```python
from build123d import *

# Parameters (mm, degrees)
SKETCH1_R               = 9
SKETCH1_W               = 9.9
SKETCH1_H               = 9.9
BOSS_EXTRUDE1_DEPTH     = 10
SKETCH2_R               = 17.5
BOSS_EXTRUDE2_DEPTH     = 6.5
CUT_EXTRUDE1_REACH      = 28.693
SKETCH3_R               = 1.25
CUT_EXTRUDE2_DEPTH      = 30.744747435
CUT_EXTRUDE2_DEPTH_BACK = 30.744747435
SKETCH4_R               = 1.5
CUT_EXTRUDE3_DEPTH      = 10
CUT_EXTRUDE3_DEPTH_BACK = 10
SKETCH6_W               = 9.9
SKETCH6_H               = 9.9
SKETCH8_W               = 5.75
SKETCH8_H               = 2.75
CUT_EXTRUDE4_DEPTH      = 5
CUT_EXTRUDE5_DEPTH      = 2.75
CIRPATTERN1_START       = 11.875
CIRPATTERN1_OUTLINE_R   = 1.25
CIRPATTERN1_DEPTH       = 2.75


# Read off the part's stored shape, not the designer's step: CirPattern1
with BuildPart() as part:
    # Sketch1 → Boss-Extrude1 (new body)
    with BuildSketch(Plane(origin=(0, 0, 0), x_dir=(1, 0, 0), z_dir=(0, 1, 0))):
        with Locations(Location((0, 0, 0), (0, 0, 270))):
            Circle(SKETCH1_R)
        Rectangle(SKETCH1_W, SKETCH1_H, mode=Mode.SUBTRACT)
    extrude(amount=BOSS_EXTRUDE1_DEPTH)

    # Sketch2 → Boss-Extrude2 (add)
    with BuildSketch(Plane(origin=(0, 10, 0), x_dir=(1, 0, 0), z_dir=(0, 1, 0))):
        with Locations(Location((0, 0, 0), (0, 0, 90))):
            Circle(SKETCH2_R)
    extrude(amount=BOSS_EXTRUDE2_DEPTH)

    # Sketch3 → Cut-Extrude1 (cut, up to next)
    with BuildSketch(Plane.XZ.offset(-10), mode=Mode.PRIVATE) as cut_extrude1_sk1:
        with Locations(Location((12.1, 0, 0), (0, 0, 270))):
            Circle(SKETCH3_R)
    cut_extrude1_tool1 = extrude(cut_extrude1_sk1.sketch, amount=-CUT_EXTRUDE1_REACH, mode=Mode.PRIVATE) & part.part
    # Sketch3 → Cut-Extrude1 (cut, up to next)
    with BuildSketch(Plane.XZ.offset(-10), mode=Mode.PRIVATE) as cut_extrude1_sk2:
        with Locations(Location((0, -12.1, 0), (0, 0, 270))):
            Circle(SKETCH3_R)
    cut_extrude1_tool2 = extrude(cut_extrude1_sk2.sketch, amount=-CUT_EXTRUDE1_REACH, mode=Mode.PRIVATE) & part.part
    # Sketch3 → Cut-Extrude1 (cut, up to next)
    with BuildSketch(Plane.XZ.offset(-10), mode=Mode.PRIVATE) as cut_extrude1_sk3:
        with Locations(Location((-12.1, 0, 0), (0, 0, 270))):
            Circle(SKETCH3_R)
    cut_extrude1_tool3 = extrude(cut_extrude1_sk3.sketch, amount=-CUT_EXTRUDE1_REACH, mode=Mode.PRIVATE) & part.part
    # Sketch3 → Cut-Extrude1 (cut, up to next)
    with BuildSketch(Plane.XZ.offset(-10), mode=Mode.PRIVATE) as cut_extrude1_sk4:
        with Locations(Location((0, 12.1, 0), (0, 0, 270))):
            Circle(SKETCH3_R)
    cut_extrude1_tool4 = extrude(cut_extrude1_sk4.sketch, amount=-CUT_EXTRUDE1_REACH, mode=Mode.PRIVATE) & part.part
    add(cut_extrude1_tool1.solids().sort_by_distance((12.1, 10, 0))[0], mode=Mode.SUBTRACT)
    add(cut_extrude1_tool2.solids().sort_by_distance((0, 10, -12.1))[0], mode=Mode.SUBTRACT)
    add(cut_extrude1_tool3.solids().sort_by_distance((-12.1, 10, 0))[0], mode=Mode.SUBTRACT)
    add(cut_extrude1_tool4.solids().sort_by_distance((0, 10, 12.1))[0], mode=Mode.SUBTRACT)

    # Sketch4 → Cut-Extrude2 (cut, two sides: drawn at the far end of the back side and taken through both)
    with BuildSketch(Plane.XY.offset(-CUT_EXTRUDE2_DEPTH_BACK)):
        with Locations((0, 4.916404418)):
            Circle(SKETCH4_R)
    extrude(amount=CUT_EXTRUDE2_DEPTH + CUT_EXTRUDE2_DEPTH_BACK, mode=Mode.SUBTRACT)

    # Sketch6 → Cut-Extrude3 (cut, two sides: drawn at the far end of the back side and taken through both)
    with BuildSketch(Plane(origin=(0, 10, 0), x_dir=(-1, 0, 0), z_dir=(0, -1, 0)).offset(-CUT_EXTRUDE3_DEPTH_BACK)):
        Rectangle(SKETCH6_W, SKETCH6_H)
    extrude(amount=CUT_EXTRUDE3_DEPTH + CUT_EXTRUDE3_DEPTH_BACK, mode=Mode.SUBTRACT)

    # Sketch8 → Cut-Extrude4 (cut)
    with BuildSketch(Plane(origin=(17.5, 0, 0), x_dir=(0, 0, -1), z_dir=(1, 0, 0))):
        with Locations((0, 13.25)):
            Rectangle(SKETCH8_W, SKETCH8_H)
    extrude(amount=-CUT_EXTRUDE4_DEPTH, mode=Mode.SUBTRACT)

    # Sketch9 → Cut-Extrude5 (cut)
    with BuildSketch(Plane.XZ.offset(-14.625)):
        Polygon((15.419764048, 0), (13.759882024, 2.875), (10.440117976, 2.875), (8.780235952, 0), (10.440117976, -2.875), (13.759882024, -2.875), align=None)
    extrude(amount=CUT_EXTRUDE5_DEPTH, mode=Mode.SUBTRACT)

    # CirPattern1 outline → CirPattern1 (cut)
    # profile 1 of 3: a face of its own
    with BuildSketch(Plane(origin=(0, 0, 0), x_dir=(1, 0, 0), z_dir=(0, 1, 0)).offset(CIRPATTERN1_START)):
        with BuildLine():
            Line((-8.780235952, 0), (-10.440117976, 2.875))
            Line((-10.440117976, 2.875), (-17.26222393, 2.875))
            ThreePointArc((-17.26222393, 2.875), (-17.5, 0), (-17.26222393, -2.875))
            Line((-17.26222393, -2.875), (-10.440117976, -2.875))
            Line((-10.440117976, -2.875), (-8.780235952, 0))
        make_face()
        with Locations((-12.1, 0)):
            Circle(CIRPATTERN1_OUTLINE_R, mode=Mode.SUBTRACT)
    # profile 2 of 3: a face of its own
    with BuildSketch(Plane(origin=(0, 0, 0), x_dir=(1, 0, 0), z_dir=(0, 1, 0)).offset(CIRPATTERN1_START)):
        with BuildLine():
            ThreePointArc((2.875, 17.26222393), (0, 17.5), (-2.875, 17.26222393))
            Line((-2.875, 17.26222393), (-2.875, 10.440117976))
            Line((-2.875, 10.440117976), (0, 8.780235952))
            Line((0, 8.780235952), (2.875, 10.440117976))
            Line((2.875, 10.440117976), (2.875, 17.26222393))
        make_face()
        with Locations((0, 12.1)):
            Circle(CIRPATTERN1_OUTLINE_R, mode=Mode.SUBTRACT)
    # profile 3 of 3: a face of its own
    with BuildSketch(Plane(origin=(0, 0, 0), x_dir=(1, 0, 0), z_dir=(0, 1, 0)).offset(CIRPATTERN1_START)):
        with BuildLine():
            Line((-2.875, -10.440117976), (-2.875, -17.26222393))
            ThreePointArc((-2.875, -17.26222393), (0, -17.5), (2.875, -17.26222393))
            Line((2.875, -17.26222393), (2.875, -10.440117976))
            Line((2.875, -10.440117976), (0, -8.780235952))
            Line((0, -8.780235952), (-2.875, -10.440117976))
        make_face()
        with Locations((0, -12.1)):
            Circle(CIRPATTERN1_OUTLINE_R, mode=Mode.SUBTRACT)
    extrude(amount=CIRPATTERN1_DEPTH, mode=Mode.SUBTRACT)


solid = part.part
```
CAD build for the part. Positions are in the model's coordinates, mm. A direction names the side the tool comes from. Round coordinates to 2 decimals unless told otherwise and drop trailing zeros. Loops run counter-clockwise (first coordinate to the right, second up) from the corner with the lowest first, then second, coordinate; pieces in that order, holes last. Notation, with made-up numbers: M 56,14.5 L 93,14.5 A20 ccw 93,41.5 Z; hole C 43,-23 d1. An arc over 180 degrees is marked long. Return JSON: item names as keys, results as strings. Group by question number.
(1) Saw through at A-A, the plane y = 12.5. List the corners of the cut face in (x, z) (3 decimals).
(2) Wall check: probe 1 along X at (y, z) = (2.25, 0); probe 2 along Y at (x, z) = (2.5, 14) (3 decimals); probe 3 along Y at (x, z) = (-6, -14). Give the ranges that are in metal, low to high. Write a range as [from, to].
(3) Saw through at D-D, the plane y = 7.5. List the corners of the cut face in (x, z), and give its area (3 significant figures).
(4) Tool access for faces 1 (the flat face through (14, 11.875, 0)), 2 (the flat face through (0, 14.625, -14)), 3 (the flat face through (2.875, 13, 14)): list every direction of +Z, -Z, +X, -X, +Y, -Y with a clear straight run to the whole face (end or side of a thin tool).
(5) Saw through at C-C, the plane z = -2. List the corners of the cut face in (x, y) (3 decimals), and give its area (3 significant figures).
(6) Mould opens along Z. For faces 4 (the flat face through (-1.42, 13.23, 9.6)), 5 (the flat face through (0, 11.875, 14)), 6 (the cylindrical face through (0.38, 15.55, -13.29)) say: +Z half, -Z half, draft (parallel to the pull), parting line (faces both ways), or undercut.
(7) Saw through at B-B, the plane x = 12.1. List the corners of the cut face in (y, z) (3 decimals).
(8) Drop flat-ended pins along their axis: P1, Ø3, axis at x = 0, z = -12.1, coming from the +Y side; P2, Ø2, axis at x = 0, z = 12.1, coming from the -Y side; P3, Ø3, axis at y = 11.5, z = 12.5, coming from the +X side; P4, Ø1.4, axis at y = 13, z = -15.5, coming from the +X side. Give the stop position or say it passes through.
Answer list:
{
 "1": {"outline": "M -17.262,-2.875 A17.5 ccw -2.875,-17.262 L -2.875,-10.44 L 0,-8.78 L 2.875,-10.44 L 2.875,-17.262 A17.5 ccw 17.262,-2.875 L 10.44,-2.875 L 8.78,0 L 10.44,2.875 L 17.262,2.875 A17.5 ccw 2.875,17.262 L 2.875,10.44 L 0,8.78 L -2.875,10.44 L -2.875,17.262 A17.5 ccw -17.262,2.875 L -10.44,2.875 L -8.78,0 L -10.44,-2.875 Z; hole M -4.95,-4.95 L 4.95,-4.95 L 4.95,4.95 L -4.95,4.95 Z"},
 "2": {"probe 1": "[-9, -4.95], [4.95, 9]", "probe 2": "[10, 11.875], [14.625, 16.5]", "probe 3": "[10, 16.5]"},
 "3": {"outline": "C 0,0 d18; hole M -4.95,-4.95 L 4.95,-4.95 L 4.95,4.95 L -4.95,4.95 Z", "area": "156 mm2"},
 "4": {"face 1": "+X", "face 2": "-Z", "face 3": "+Z"},
 "5": {"outline": "M -17.385,10 L -8.775,10 L -8.775,0 L -4.95,0 L -4.95,16.5 L -17.385,16.5 L -17.385,14.625 L -9.935,14.625 L -9.935,11.875 L -17.385,11.875 Z; M 4.95,0 L 8.775,0 L 8.775,10 L 17.385,10 L 17.385,11.875 L 9.935,11.875 L 9.935,14.625 L 17.385,14.625 L 17.385,16.5 L 4.95,16.5 Z", "area": "197 mm2"},
 "6": {"face 4": "+Z half", "face 5": "draft", "face 6": "undercut"},
 "7": {"outline": "M 10,-12.643 L 16.5,-12.643 L 16.5,-1.25 L 14.625,-1.25 L 14.625,-2.875 L 11.875,-2.875 L 11.875,-1.25 L 10,-1.25 Z; M 10,1.25 L 11.875,1.25 L 11.875,2.875 L 14.625,2.875 L 14.625,1.25 L 16.5,1.25 L 16.5,12.643 L 10,12.643 Z"},
 "8": {"P1": "y = 16.5", "P2": "through", "P3": "x = 13.61", "P4": "x = 9.34"}
}
